Can you work these out from the model? Positions are in its coordinate system, mm. Face numbers are marked on the shaded views. Give positions to 0.01 mm unless a question says otherwise; leave off trailing zeros. Loops run counter-clockwise (first coordinate to the right, second up) from the corner with the lowest first, then second, coordinate; pieces in that order, holes last. Notation, with made-up numbers: M 32.25,44.5 L 65.25,44.5 A32 ccw 65.25,79.5 Z; hole C 9.5,1.5 d8. An arc over 180 degrees is marked long. Put each result on its own line as item: value. Start each with the question number.
1) If we mould it in two halves opening along X, with no side actions, what happens to the marked faces 1, 2 and 3? For each: +X half, -X half, draft (parallel to the pull), parting line (faces both ways), or undercut.
2) Imagine slicing it at B-B (z = 1.3). State how many separate pieces and enclosed holes the cut face has, then the cut area to 3 significant figures.
3) Please list where these lines run through material, in increasing order: line 1 along Z through (x, y) = (-4, 5.5); line 2 along Y through (x, z) = (2, 0.4). Write a range as from..to.
4) Imagine slicing it at A-A (x = -1.25). Write out the boundary of the cut face in (y, z), then the cut area to 3 significant figures.
from build123d import *

# Parameters (mm, degrees)
SKETCH1_W            = 25.908
SKETCH1_H            = 8.001
BOSS_EXTRUDE1_DEPTH  = 4.953
SKETCH2_W            = 0.7874
SKETCH2_H            = 0.7874
CUT_EXTRUDE1_DEPTH   = 9.001
LPATTERN1_COUNT      = 2
LPATTERN1_PITCH      = 2.54
LPATTERN1_COUNT_DIR2 = 10
LPATTERN1_PITCH_DIR2 = 2.54
SKETCH3_W            = 0.508
SKETCH3_H            = 4.953
BOSS_EXTRUDE2_DEPTH  = 0.508
LPATTERN2_COUNT      = 11
LPATTERN2_PITCH      = 2.54


with BuildPart() as part:
    # Sketch1 → Boss-Extrude1 (new body)
    with BuildSketch(Plane.XY.offset(2.4765)):
        with Locations((0, 4.5085)):
            Rectangle(SKETCH1_W, SKETCH1_H)
    extrude(amount=-BOSS_EXTRUDE1_DEPTH)

    # Sketch2 → Cut-Extrude1 (cut, through all)
    with BuildSketch(Plane.XZ.offset(-0.508)):
        with Locations((11.43, -1.27)):
            Rectangle(SKETCH2_W, SKETCH2_H)
    cut_extrude1 = extrude(amount=-CUT_EXTRUDE1_DEPTH, mode=Mode.SUBTRACT)

    # LPattern1: Cut-Extrude1 2 × 10
    with Locations(*[(-j * LPATTERN1_PITCH_DIR2, 0, i * LPATTERN1_PITCH) for i in range(LPATTERN1_COUNT) for j in range(LPATTERN1_COUNT_DIR2) if (i, j) != (0, 0)]):
        add(cut_extrude1, mode=Mode.SUBTRACT)

    # Sketch3 → Boss-Extrude2 (add)
    with BuildSketch(Plane.XZ.offset(-0.508)):
        with Locations((-12.7, 0)):
            Rectangle(SKETCH3_W, SKETCH3_H)
    boss_extrude2 = extrude(amount=BOSS_EXTRUDE2_DEPTH)

    # LPattern2: Boss-Extrude2 ×11
    with Locations(*[(i * LPATTERN2_PITCH, 0, 0) for i in range(1, LPATTERN2_COUNT)]):
        add(boss_extrude2)


solid = part.part
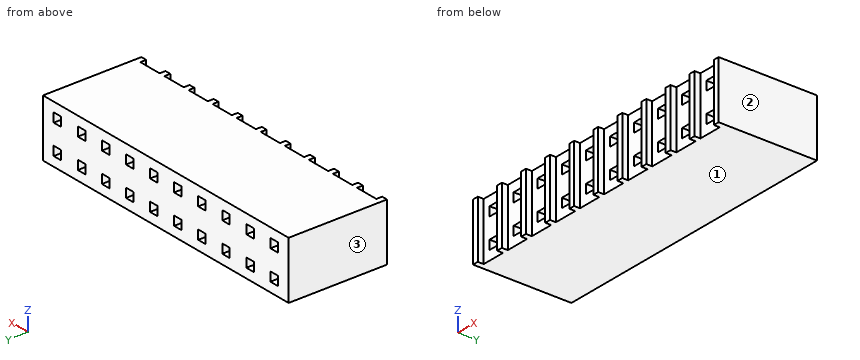
Recorded:
1. face 1: draft
1. face 2: +X half
1. face 3: -X half
2. separate pieces: 11
2. enclosed holes: 0
2. area: 147 mm²
3. line 1: -2.48..-1.66, -0.88..0.88, 1.66..2.48
3. line 2: 0.51..8.51
4. outline: M 0.51,-2.48 L 8.51,-2.48 L 8.51,-1.66 L 0.51,-1.66 Z; M 0.51,-0.88 L 8.51,-0.88 L 8.51,0.88 L 0.51,0.88 Z; M 0.51,1.66 L 8.51,1.66 L 8.51,2.48 L 0.51,2.48 Z
4. area: 27.0 mm²
